Verification items for the finished model (mm, model axes). Face numbers are marked on the shaded views. A direction names the side the tool comes from. Give positions to 0.01 mm unless a question says otherwise; leave off trailing zeros. Loops run counter-clockwise (first coordinate to the right, second up) from the corner with the lowest first, then second, coordinate; pieces in that order, holes last. Notation, with made-up numbers: (-32, -22) -> (-18, -22) arc R17 cw to (-18, -2) -> close; hole circle Ø10 at (23.25, 1). An arc over 180 degrees is marked (long way). Use one line per item in the form item = value. Start each with the question number.
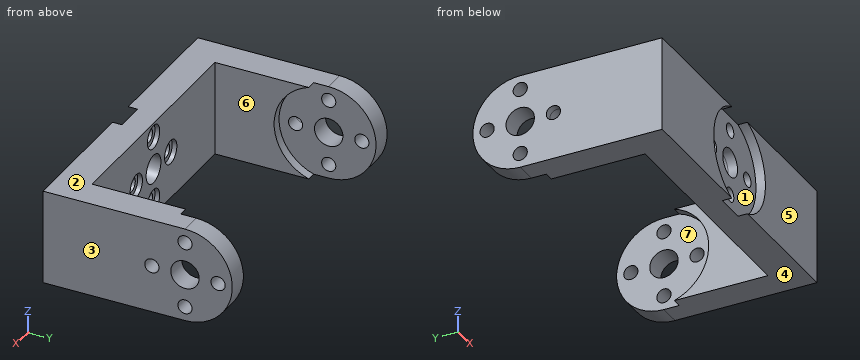
from build123d import *

# Parameters (mm, degrees)
CROQUIS1_W                  = 50
CROQUIS1_H                  = 20
CROQUIS1_R                  = 3
SALIENTE_EXTRUIR1_DEPTH     = 5
CROQUIS2_R                  = 10.5
CORTAR_EXTRUIR7_DEPTH       = 2
CROQUIS7_R                  = 1.5
CORTAR_EXTRUIR8_DEPTH       = 4
CROQUIS8_R                  = 2.5
CORTAR_EXTRUIR9_DEPTH       = 1
CROQUIS9_W                  = 5
CROQUIS9_H                  = 20
SALIENTE_EXTRUIR3_DEPTH     = 33
CROQUIS10_R                 = 3
CORTAR_EXTRUIR10_DEPTH      = 50
CROQUIS11_R                 = 10.5
CORTAR_EXTRUIR11_DEPTH      = 42
CORTAR_EXTRUIR11_DEPTH_BACK = 2
CROQUIS12_R                 = 1.5
CORTAR_EXTRUIR12_DEPTH      = 50
CORTAR_EXTRUIR12_DEPTH_BACK = 6
CROQUIS13_R                 = 1.5
CROQUIS13_R_2               = 3
SALIENTE_EXTRUIR4_DEPTH     = 5
CROQUIS14_R                 = 1.5
CROQUIS14_R_2               = 3
SALIENTE_EXTRUIR5_DEPTH     = 5
CORTAR_EXTRUIR14_DEPTH      = 45
CORTAR_EXTRUIR14_DEPTH_BACK = 5
CORTAR_EXTRUIR15_DEPTH      = 49
CORTAR_EXTRUIR15_DEPTH_BACK = 5
SALIENTE_EXTRUIR6_DEPTH     = 2
CROQUIS18_R                 = 3
CROQUIS18_R_2               = 1.5
SALIENTE_EXTRUIR7_DEPTH     = 2
CROQUIS19_R                 = 1.5
CROQUIS19_R_2               = 3
SALIENTE_EXTRUIR8_DEPTH     = 1.5
CROQUIS20_R                 = 1.5
CROQUIS20_R_2               = 3
SALIENTE_EXTRUIR9_DEPTH     = 1.5


with BuildPart() as part:
    # Croquis1 → Saliente-Extruir1 (new body)
    with BuildSketch(Plane(origin=(0, 0, 0), x_dir=(1, 0, 0), z_dir=(0, 1, 0))):
        Rectangle(CROQUIS1_W, CROQUIS1_H)
        Circle(CROQUIS1_R, mode=Mode.SUBTRACT)
    extrude(amount=SALIENTE_EXTRUIR1_DEPTH)

    # Croquis2 → Cortar-Extruir7 (cut)
    with BuildSketch(Plane.XZ):
        Circle(CROQUIS2_R)
    extrude(amount=-CORTAR_EXTRUIR7_DEPTH, mode=Mode.SUBTRACT)

    # Croquis7 → Cortar-Extruir8 (cut)
    with BuildSketch(Plane.XZ.offset(-2)):
        with Locations((0, 7)):
            Circle(CROQUIS7_R)
        with Locations((7, 0)):
            Circle(CROQUIS7_R)
        with Locations((0, -7)):
            Circle(CROQUIS7_R)
        with Locations((-7, 0)):
            Circle(CROQUIS7_R)
    extrude(amount=-CORTAR_EXTRUIR8_DEPTH, mode=Mode.SUBTRACT)

    # Croquis8 → Cortar-Extruir9 (cut)
    with BuildSketch(Plane(origin=(0, 5, 0), x_dir=(1, 0, 0), z_dir=(0, 1, 0))):
        with Locations((0, 7)):
            Circle(CROQUIS8_R)
        with Locations((7, 0)):
            Circle(CROQUIS8_R)
        with Locations((0, -7)):
            Circle(CROQUIS8_R)
        with Locations((-7, 0)):
            Circle(CROQUIS8_R)
    extrude(amount=-CORTAR_EXTRUIR9_DEPTH, mode=Mode.SUBTRACT)

    # Croquis9 → Saliente-Extruir3 (add)
    with BuildSketch(Plane(origin=(0, 5, 0), x_dir=(1, 0, 0), z_dir=(0, 1, 0))):
        with Locations((22.5, 0)):
            Rectangle(CROQUIS9_W, CROQUIS9_H)
        with Locations((-22.5, 0)):
            Rectangle(CROQUIS9_W, CROQUIS9_H)
    extrude(amount=SALIENTE_EXTRUIR3_DEPTH)

    # Croquis10 → Cortar-Extruir10 (cut)
    with BuildSketch(Plane(origin=(25, 0, 0), x_dir=(0, 0, -1), z_dir=(1, 0, 0))):
        with Locations((0, 28)):
            Circle(CROQUIS10_R)
        with BuildLine():
            Line((10, 28), (21.898985217, 31.221805306))
            Line((21.898985217, 31.221805306), (12.889165909, 40.913504361))
            Line((12.889165909, 40.913504361), (-22.207421629, 40.012243034))
            Line((-22.207421629, 40.012243034), (-10, 28))
            ThreePointArc((-10, 28), (0, 38), (10, 28))
        make_face()
    extrude(amount=-CORTAR_EXTRUIR10_DEPTH, mode=Mode.SUBTRACT)

    # Croquis11 → Cortar-Extruir11 (cut, two sides)
    with BuildSketch(Plane(origin=(-20, 0, 0), x_dir=(0, 0, -1), z_dir=(1, 0, 0))) as cortar_extruir11_sk:
        with Locations((0, 28)):
            Circle(CROQUIS11_R)
    extrude(amount=CORTAR_EXTRUIR11_DEPTH, mode=Mode.SUBTRACT)
    extrude(cortar_extruir11_sk.sketch, amount=-CORTAR_EXTRUIR11_DEPTH_BACK, mode=Mode.SUBTRACT)

    # Croquis12 → Cortar-Extruir12 (cut, two sides)
    with BuildSketch(Plane(origin=(-22, 0, 0), x_dir=(0, 0, -1), z_dir=(1, 0, 0))) as cortar_extruir12_sk:
        with Locations((0, 35)):
            Circle(CROQUIS12_R)
        with Locations((7, 28)):
            Circle(CROQUIS12_R)
        with Locations((0, 21)):
            Circle(CROQUIS12_R)
        with Locations((-7, 28)):
            Circle(CROQUIS12_R)
    extrude(amount=CORTAR_EXTRUIR12_DEPTH, mode=Mode.SUBTRACT)
    extrude(cortar_extruir12_sk.sketch, amount=-CORTAR_EXTRUIR12_DEPTH_BACK, mode=Mode.SUBTRACT)

    # Croquis13 → Saliente-Extruir4 (add)
    with BuildSketch(Plane(origin=(25, 0, 0), x_dir=(0, 0, -1), z_dir=(1, 0, 0))):
        with BuildLine():
            Line((10, 0), (10, 28))
            ThreePointArc((10, 28), (0, 38), (-10, 28))
            Line((-10, 28), (-10, 0))
            Line((-10, 0), (10, 0))
        make_face()
        with Locations((-7, 28)):
            Circle(CROQUIS13_R, mode=Mode.SUBTRACT)
        with Locations((0, 28)):
            Circle(CROQUIS13_R_2, mode=Mode.SUBTRACT)
        with Locations((7, 28)):
            Circle(CROQUIS13_R, mode=Mode.SUBTRACT)
        with Locations((0, 35)):
            Circle(CROQUIS13_R, mode=Mode.SUBTRACT)
        with Locations((0, 21)):
            Circle(CROQUIS13_R, mode=Mode.SUBTRACT)
    extrude(amount=SALIENTE_EXTRUIR4_DEPTH)

    # Croquis14 → Saliente-Extruir5 (add)
    with BuildSketch(Plane.ZY.offset(25)):
        with BuildLine():
            Line((10, 0), (10, 28))
            ThreePointArc((10, 28), (0, 38), (-10, 28))
            Line((-10, 28), (-10, 0))
            Line((-10, 0), (10, 0))
        make_face()
        with Locations((0, 21)):
            Circle(CROQUIS14_R, mode=Mode.SUBTRACT)
        with Locations((0, 28)):
            Circle(CROQUIS14_R_2, mode=Mode.SUBTRACT)
        with Locations((-7, 28)):
            Circle(CROQUIS14_R, mode=Mode.SUBTRACT)
        with Locations((0, 35)):
            Circle(CROQUIS14_R, mode=Mode.SUBTRACT)
        with Locations((7, 28)):
            Circle(CROQUIS14_R, mode=Mode.SUBTRACT)
    extrude(amount=SALIENTE_EXTRUIR5_DEPTH)

    # Croquis15 → Cortar-Extruir14 (cut, two sides)
    with BuildSketch(Plane(origin=(-20, 0, 0), x_dir=(0, 0, -1), z_dir=(1, 0, 0))) as cortar_extruir14_sk:
        with BuildLine():
            Line((-10, 24.798437881), (-10, 5))
            Line((-10, 5), (10, 5))
            Line((10, 5), (10, 24.798437881))
            ThreePointArc((10, 24.798437881), (0, 17.5), (-10, 24.798437881))
        make_face()
    extrude(amount=CORTAR_EXTRUIR14_DEPTH, mode=Mode.SUBTRACT)
    extrude(cortar_extruir14_sk.sketch, amount=-CORTAR_EXTRUIR14_DEPTH_BACK, mode=Mode.SUBTRACT)

    # Croquis16 → Cortar-Extruir15 (cut, two sides)
    with BuildSketch(Plane(origin=(-22, 0, 0), x_dir=(0, 0, -1), z_dir=(1, 0, 0))) as cortar_extruir15_sk:
        with BuildLine():
            Line((-10, 28), (-10, 24.798437881))
            ThreePointArc((-10, 24.798437881), (0, 17.5), (10, 24.798437881))
            Line((10, 24.798437881), (10, 28))
            ThreePointArc((10, 28), (0, 38), (-10, 28))
        make_face()
    extrude(amount=CORTAR_EXTRUIR15_DEPTH, mode=Mode.SUBTRACT)
    extrude(cortar_extruir15_sk.sketch, amount=-CORTAR_EXTRUIR15_DEPTH_BACK, mode=Mode.SUBTRACT)

    # Croquis17 → Saliente-Extruir6 (add)
    with BuildSketch(Plane.XZ):
        with BuildLine():
            Line((30, 10), (3.201562119, 10))
            ThreePointArc((3.201562119, 10), (10.5, 0), (3.201562119, -10))
            Line((3.201562119, -10), (30, -10))
            Line((30, -10), (30, 10))
        make_face()
        with BuildLine():
            Line((-30, -10), (-3.201562119, -10))
            ThreePointArc((-3.201562119, -10), (-10.5, 0), (-3.201562119, 10))
            Line((-3.201562119, 10), (-30, 10))
            Line((-30, 10), (-30, -10))
        make_face()
    extrude(amount=SALIENTE_EXTRUIR6_DEPTH)

    # Croquis18 → Saliente-Extruir7 (add)
    with BuildSketch(Plane.XZ.offset(-2)):
        with BuildLine():
            Line((3.201562119, 10), (-3.201562119, 10))
            ThreePointArc((-3.201562119, 10), (-10.5, 0), (-3.201562119, -10))
            Line((-3.201562119, -10), (3.201562119, -10))
            ThreePointArc((3.201562119, -10), (10.5, 0), (3.201562119, 10))
        make_face()
        Circle(CROQUIS18_R, mode=Mode.SUBTRACT)
        with Locations((7, 0)):
            Circle(CROQUIS18_R_2, mode=Mode.SUBTRACT)
        with Locations((0, 7)):
            Circle(CROQUIS18_R_2, mode=Mode.SUBTRACT)
        with Locations((-7, 0)):
            Circle(CROQUIS18_R_2, mode=Mode.SUBTRACT)
        with Locations((0, -7)):
            Circle(CROQUIS18_R_2, mode=Mode.SUBTRACT)
    extrude(amount=SALIENTE_EXTRUIR7_DEPTH)

    # Croquis19 → Saliente-Extruir8 (add)
    with BuildSketch(Plane(origin=(30, 0, 0), x_dir=(0, 0, -1), z_dir=(1, 0, 0))):
        with BuildLine():
            Line((-10, 28), (-10, -2))
            Line((-10, -2), (10, -2))
            Line((10, -2), (10, 28))
            ThreePointArc((10, 28), (0, 38), (-10, 28))
        make_face()
        with Locations((7, 28)):
            Circle(CROQUIS19_R, mode=Mode.SUBTRACT)
        with Locations((0, 21)):
            Circle(CROQUIS19_R, mode=Mode.SUBTRACT)
        with Locations((0, 28)):
            Circle(CROQUIS19_R_2, mode=Mode.SUBTRACT)
        with Locations((-7, 28)):
            Circle(CROQUIS19_R, mode=Mode.SUBTRACT)
        with Locations((0, 35)):
            Circle(CROQUIS19_R, mode=Mode.SUBTRACT)
    extrude(amount=SALIENTE_EXTRUIR8_DEPTH)

    # Croquis20 → Saliente-Extruir9 (add)
    with BuildSketch(Plane.ZY.offset(30)):
        with BuildLine():
            Line((-10, 28), (-10, -2))
            Line((-10, -2), (10, -2))
            Line((10, -2), (10, 28))
            ThreePointArc((10, 28), (0, 38), (-10, 28))
        make_face()
        with Locations((0, 21)):
            Circle(CROQUIS20_R, mode=Mode.SUBTRACT)
        with Locations((0, 28)):
            Circle(CROQUIS20_R_2, mode=Mode.SUBTRACT)
        with Locations((7, 28)):
            Circle(CROQUIS20_R, mode=Mode.SUBTRACT)
        with Locations((0, 35)):
            Circle(CROQUIS20_R, mode=Mode.SUBTRACT)
        with Locations((-7, 28)):
            Circle(CROQUIS20_R, mode=Mode.SUBTRACT)
    extrude(amount=SALIENTE_EXTRUIR9_DEPTH)


solid = part.part
Item 1: Draft check along Z on the marked faces 1, 2, 3 and 4. Enter one of: +Z half, -Z half, draft (parallel to the pull), parting line (faces both ways), or undercut.
Item 2: Sectioned sample at D-D, the plane y = 21. Enter the section's corners in (x, z).
Item 3: Tool access check on the marked faces 5, 6 and 7. Record the directions out of +Z, -Z, +X, -X, +Y, -Y that give a thin tool (end or side, any length) a straight path to the whole face; none if there is none.
Item 4: Sectioned sample at A-A, the plane x = 0. Enter the section's corners in (y, z).
Item 5: Material ranges on line 1 (Y direction, x = 28, z = 0); line 2 (X direction, y = 33, z = -6); line 3 (X direction, y = 14, z = 4.75), recorded low to high.
Item 6: Gauge pin test, flat ends, axial feed: pin 1 Ø5.5 at (x, z) = (8, 0) entering from +Y; pin 2 Ø8 at (x, z) = (0, 0) entering from -Y; pin 3 Ø1.5 at (x, z) = (-1, -8) entering from +Y. Record the tip position at first contact, or that the pin passes through.
Item 7: Sectioned sample at C-C, the plane z = -7. State how many separate pieces and enclosed holes the cut face has, and give its area (3 significant figures).
Item 8: Sectioned sample at B-B, the plane y = 10.5. Enter the section's corners in (x, z).
Outcome:
q1.face_1 = undercut
q1.face_2 = +Z half
q1.face_3 = draft
q1.face_4 = -Z half
q2.outline = (-31.5, -10) -> (-25, -10) -> (-25, -7.83) -> (-27, -7.83) -> (-27, -1.5) -> (-31.5, -1.5) -> close; (-31.5, 1.5) -> (-27, 1.5) -> (-27, 7.83) -> (-25, 7.83) -> (-25, 10) -> (-31.5, 10) -> close; (25, -10) -> (31.5, -10) -> (31.5, -1.5) -> (27, -1.5) -> (27, -7.83) -> (25, -7.83) -> close; (25, 7.83) -> (27, 7.83) -> (27, 1.5) -> (31.5, 1.5) -> (31.5, 10) -> (25, 10) -> close
q3.face_5 = +Z, -Z, +X, -X, -Y
q3.face_6 = +Z, -Z, +Y
q3.face_7 = +Y
q4.outline = (0, -10) -> (5, -10) -> (5, -9.5) -> (4, -9.5) -> (4, -8.5) -> (0, -8.5) -> close; (0, -5.5) -> (4, -5.5) -> (4, -4.5) -> (5, -4.5) -> (5, -3) -> (0, -3) -> close; (0, 3) -> (5, 3) -> (5, 4.5) -> (4, 4.5) -> (4, 5.5) -> (0, 5.5) -> close; (0, 8.5) -> (4, 8.5) -> (4, 9.5) -> (5, 9.5) -> (5, 10) -> (0, 10) -> close
q5.line_1 = -2 to 19.5, 22.5 to 25, 31 to 33.5, 36.5 to 38
q5.line_2 = -31.5 to -27, 27 to 31.5
q5.line_3 = -31.5 to -25, 25 to 31.5
q6.pin_1 = 5
q6.pin_2 = 0
q6.pin_3 = 4
q7.separate_pieces = 4
q7.enclosed_holes = 0
q7.area = 698 mm^2
q8.outline = (-31.5, -10) -> (-25, -10) -> (-25, 10) -> (-31.5, 10) -> close; (25, -10) -> (31.5, -10) -> (31.5, 10) -> (25, 10) -> close
